```python
from build123d import *

# Parameters (mm, degrees)
EXTRUDE_1_DEPTH     = 10
SKETCH_2_R          = 5
EXTRUDE_2_DEPTH     = 6
SKETCH_3_R          = 6
EXTRUDE_3_DEPTH     = 1
SKETCH_4_R          = 1.8
CUT_EXTRUDE_1_DEPTH = 38.549966711
FILLET_1_R          = 1


with BuildPart() as part:
    # ｽｹｯﾁ1 → ﾎﾞｽ - 押し出し1 (new body)
    with BuildSketch(Plane(origin=(0, 0, 0), x_dir=(1, 0, 0), z_dir=(0, 1, 0))):
        with BuildLine():
            Line((-8, 0), (-8, 10))
            Line((-8, 10), (-25, 10))
            Line((-25, 10), (-25, 15))
            Line((-25, 15), (25, 15))
            Line((25, 15), (25, 10))
            Line((25, 10), (8, 10))
            Line((8, 10), (8, 0))
            ThreePointArc((8, 0), (0, -8), (-8, 0))
        make_face()
    extrude(amount=EXTRUDE_1_DEPTH)

    # ｽｹｯﾁ2 → ﾎﾞｽ - 押し出し2 (add)
    with BuildSketch(Plane(origin=(0, 10, 0), x_dir=(1, 0, 0), z_dir=(0, 1, 0))):
        with Locations(Location((0, 0, 0), (0, 0, 270))):
            Circle(SKETCH_2_R)
    extrude(amount=EXTRUDE_2_DEPTH)

    # ｽｹｯﾁ3 → ﾎﾞｽ - 押し出し3 (add)
    with BuildSketch(Plane(origin=(0, 10, 0), x_dir=(1, 0, 0), z_dir=(0, 1, 0))):
        with Locations(Location((0, 0, 0), (0, 0, 270))):
            Circle(SKETCH_3_R)
    extrude(amount=EXTRUDE_3_DEPTH)

    # ｽｹｯﾁ4 → ｶｯﾄ - 押し出し1 (cut, through all)
    with BuildSketch(Plane(origin=(0, 0, -15), x_dir=(-1, 0, 0), z_dir=(0, 0, -1))):
        with Locations((20, 5)):
            Circle(SKETCH_4_R)
        with Locations((-20, 5)):
            Circle(SKETCH_4_R)
    extrude(amount=-CUT_EXTRUDE_1_DEPTH, mode=Mode.SUBTRACT)

    # ﾌｨﾚｯﾄ1
    fillet_1_edges = [part.edges().sort_by_distance(p)[0] for p in [
        (-8, 5, -10),
        (8, 5, -10),
    ]]
    fillet(fillet_1_edges, radius=FILLET_1_R)


solid = part.part
```
Read the model definition and answer for the solid it produces. Units are mm, in the model's axes. A direction names the side the tool comes from. Coordinates: 2 decimals unless noted, no trailing zeros. Write each loop counter-clockwise with the first axis right and the second up, starting at its lowest first coordinate (ties: lowest second). Pieces come first, ordered by that corner, then holes. Notation, with made-up numbers: (-6.75, -34) - (12.25, -34) arc R33 cw to (12.25, -4) - close; hole circle Ø1 at (57.25, 38.5). An arc over 180 degrees is marked (long way). Answer as a JSON object with one key per item and string values. Group by question number.
1. The mould has two halves that part along Y. Classify faces 6 (the flat face through (0, 0, -6)), 7 (the flat face through (0, 16, 0)), 8 (the cylindrical face through (-4.88, 13.46, -1.08)), 9 (the cylindrical face through (-19.61, 3.243, -12.535)): +Y half, -Y half, draft (parallel to the pull), parting line (faces both ways), or undercut.
2. A cutting plane is placed at C-C (x = 0). Determine the outline of the cut face in (y, z).
3. A cutting plane is placed at A-A (y = 5). Determine the outline of the cut face in (x, z), plus the area to 3 significant figures.
4. A cutting plane is placed at B-B (x = 20). Determine the outline of the cut face in (y, z).
5. Which of the six approach directions +Z, -Z, +X, -X, +Y, -Y give full straight-line access (tool end or side, diameter ignored) to faces 1 (the cylindrical face through (1.802, 10.493, 5.723)), 2 (the flat face through (-8, 5, -4)), 3 (the flat face through (-25, 5, -12)), 4 (the flat face through (17, 5, -10)), 5 (the flat face through (0, 5, -15))?
6. Consider L1, parallel to Y at x = 20, z = -13.4; L2, parallel to Y at x = 0, z = -10.5; L3, parallel to Z at x = 12.5, y = 3.75. Determine where each line is inside the solid, lowest interval first. Write a range as [from, to].
7. A cutting plane is placed at D-D (y = 7.75). Determine the outline of the cut face in (x, z).
8. Each of these flat-tipped pins is pushed along its axis until it touches: P1, Ø1, axis at y = 2, z = -3, coming from the +X side; P2, Ø1.5, axis at x = 4, y = 13, coming from the -Z side; P3, Ø1.5, axis at x = -12.5, z = -8, coming from the +Y side; P4, Ø6, axis at x = 20, y = 5, coming from the -Z side. Where does it stop, or does it pass through?
Worked out:
{
 "1": {"face 6": "-Y half", "face 7": "+Y half", "face 8": "draft", "face 9": "undercut"},
 "2": {"outline": "(0, -15) - (10, -15) - (10, -6) - (11, -6) - (11, -5) - (16, -5) - (16, 5) - (11, 5) - (11, 6) - (10, 6) - (10, 8) - (0, 8) - close"},
 "3": {"outline": "(-25, -15) - (-21.8, -15) - (-21.8, -10) - (-25, -10) - close; (-18.2, -15) - (18.2, -15) - (18.2, -10) - (9, -10) arc R1 cw to (8, -9) - (8, 0) arc R8 ccw to (-8, 0) - (-8, -9) arc R1 cw to (-9, -10) - (-18.2, -10) - close; (21.8, -15) - (25, -15) - (25, -10) - (21.8, -10) - close", "area": "475 mm²"},
 "4": {"outline": "(0, -15) - (3.2, -15) - (3.2, -10) - (0, -10) - close; (6.8, -15) - (10, -15) - (10, -10) - (6.8, -10) - close"},
 "5": {"face 1": "+Y", "face 2": "+Z, -X, +Y, -Y", "face 3": "+Z, -Z, -X, +Y, -Y", "face 4": "+Z, +X, +Y, -Y", "face 5": "-Z, +X, -X, +Y, -Y"},
 "6": {"L1": "y = [0, 3.2], [6.8, 10]", "L2": "y = [0, 10]", "L3": "z = [-15, -10]"},
 "7": {"outline": "(-25, -15) - (25, -15) - (25, -10) - (9, -10) arc R1 cw to (8, -9) - (8, 0) arc R8 ccw to (-8, 0) - (-8, -9) arc R1 cw to (-9, -10) - (-25, -10) - close"},
 "8": {"P1": "stops at x = 8", "P2": "stops at z = -3.8", "P3": "passes through", "P4": "stops at z = -15"}
}
